Read the model definition and answer for the solid it produces. Units are mm, in the model's axes. A direction names the side the tool comes from. Give positions to 0.01 mm unless a question says otherwise; leave off trailing zeros. Write each loop counter-clockwise with the first axis right and the second up, starting at its lowest first coordinate (ties: lowest second). Pieces come first, ordered by that corner, then holes. Notation, with made-up numbers: M 58.5,35.25 L 117.5,35.25 A9 cw 117.5,46.25 Z; hole C -37.5,56.25 d7. An arc over 180 degrees is marked long. Put each result on its own line as item: value.
from build123d import *

# Parameters (mm, degrees)
SKETCH2_R           = 1.5
SKETCH2_R_2         = 33
BOSS_EXTRUDE1_DEPTH = 2
CUT_EXTRUDE1_DEPTH  = 74.566296631
FILLET1_R           = 1


with BuildPart() as part:
    # Sketch2 → Boss-Extrude1 (new body)
    with BuildSketch(Plane(origin=(0, 0, 0), x_dir=(1, 0, 0), z_dir=(0, 1, 0))):
        with BuildLine():
            Line((17.897079586, 48.929734976), (40.149284407, 43.651218265))
            ThreePointArc((40.149284407, 43.651218265), (42.540265174, 42.312242187), (43.866371506, 39.91409958))
            Line((43.866371506, 39.91409958), (49.02521675, 17.633846579))
            ThreePointArc((49.02521675, 17.633846579), (49.23478351, 16.809026698), (49.479249782, 15.993868858))
            ThreePointArc((49.479249782, 15.993868858), (51.999812242, -0.139738387), (49.392575566, -16.259565766))
            ThreePointArc((49.392575566, -16.259565766), (49.143731732, -17.073397941), (48.929734976, -17.897079586))
            Line((48.929734976, -17.897079586), (43.651218265, -40.149284407))
            ThreePointArc((43.651218265, -40.149284407), (42.312242187, -42.540265174), (39.91409958, -43.866371506))
            Line((39.91409958, -43.866371506), (17.633846579, -49.02521675))
            ThreePointArc((17.633846579, -49.02521675), (16.809026698, -49.23478351), (15.993868858, -49.479249782))
            ThreePointArc((15.993868858, -49.479249782), (-0.139738387, -51.999812242), (-16.259565766, -49.392575566))
            ThreePointArc((-16.259565766, -49.392575566), (-17.073397941, -49.143731732), (-17.897079586, -48.929734976))
            Line((-17.897079586, -48.929734976), (-40.149284407, -43.651218265))
            ThreePointArc((-40.149284407, -43.651218265), (-42.540265174, -42.312242187), (-43.866371506, -39.91409958))
            Line((-43.866371506, -39.91409958), (-49.02521675, -17.633846579))
            ThreePointArc((-49.02521675, -17.633846579), (-49.23478351, -16.809026698), (-49.479249782, -15.993868858))
            ThreePointArc((-49.479249782, -15.993868858), (-51.999812242, 0.139738387), (-49.392575566, 16.259565766))
            ThreePointArc((-49.392575566, 16.259565766), (-49.143731732, 17.073397941), (-48.929734976, 17.897079586))
            Line((-48.929734976, 17.897079586), (-43.651218265, 40.149284407))
            ThreePointArc((-43.651218265, 40.149284407), (-42.312242187, 42.540265174), (-39.91409958, 43.866371506))
            Line((-39.91409958, 43.866371506), (-17.633846579, 49.02521675))
            ThreePointArc((-17.633846579, 49.02521675), (-16.809026698, 49.23478351), (-15.993868858, 49.479249782))
            ThreePointArc((-15.993868858, 49.479249782), (-8.026622704, 51.3767781), (0.139738387, 51.999812242))
            ThreePointArc((0.139738387, 51.999812242), (8.302633013, 51.332896714), (16.259565766, 49.392575566))
            ThreePointArc((16.259565766, 49.392575566), (17.073397941, 49.143731732), (17.897079586, 48.929734976))
        make_face()
        with Locations(Location((-38.8907, 38.8907, 0), (0, 0, 270))):
            Circle(SKETCH2_R, mode=Mode.SUBTRACT)
        with Locations(Location((38.8907, 38.8907, 0), (0, 0, 90))):
            Circle(SKETCH2_R, mode=Mode.SUBTRACT)
        with Locations(Location((38.8907, -38.8907, 0), (0, 0, 270))):
            Circle(SKETCH2_R, mode=Mode.SUBTRACT)
        with Locations(Location((-38.8907, -38.8907, 0), (0, 0, 90))):
            Circle(SKETCH2_R, mode=Mode.SUBTRACT)
        with Locations(Location((0, 0, 0), (0, 0, 270))):
            Circle(SKETCH2_R_2, mode=Mode.SUBTRACT)
        with Locations(Location((0, 38.8907, 0), (0, 0, 270))):
            Circle(SKETCH2_R, mode=Mode.SUBTRACT)
        with Locations(Location((-33.680334171, -19.44535, 0), (0, 0, 270))):
            Circle(SKETCH2_R, mode=Mode.SUBTRACT)
        with Locations(Location((33.680334171, -19.44535, 0), (0, 0, 270))):
            Circle(SKETCH2_R, mode=Mode.SUBTRACT)
    extrude(amount=BOSS_EXTRUDE1_DEPTH)

    # Sketch3 → Cut-Extrude1 (cut, through all)
    with BuildSketch(Plane(origin=(0, 2, 0), x_dir=(1, 0, 0), z_dir=(0, 1, 0))):
        with BuildLine():
            Line((-21.21199112, 25.279466623), (-28.925442436, 34.47199994))
            ThreePointArc((-28.925442436, 34.47199994), (-38.97114317, 22.5), (-44.316348886, 7.814167995))
            Line((-44.316348886, 7.814167995), (-32.498655849, 5.730389863))
            ThreePointArc((-32.498655849, 5.730389863), (-28.578838325, 16.5), (-21.21199112, 25.279466623))
        make_face()
    extrude(amount=-CUT_EXTRUDE1_DEPTH, mode=Mode.SUBTRACT)

    # Fillet1
    fillet1_edges = [part.edges().sort_by_distance(p)[0] for p in [
        (-44.316348886, 1, -7.814167995),
        (-28.925442436, 1, -34.47199994),
        (-21.21199112, 1, -25.279466623),
        (-32.498655849, 1, -5.730389863),
    ]]
    fillet(fillet1_edges, radius=FILLET1_R)


solid = part.part
(1) Section A-A on z = 0 is taken. Determine the outline of the cut face in (x, y).
Result:
outline: M -52,0 L -33,0 L -33,2 L -52,2 Z; M 33,0 L 52,0 L 52,2 L 33,2 Z
(2) Section C-C on y = 0.55 is taken. Give the number of separate pieces and of enclosed holes in the cut face, and give its area (3 significant figures).
Result:
separate pieces: 1
enclosed holes: 8
area: 5,340 mm²
(3) Given pin 1 Ø1 at (y, z) = (1, -14.5) entering from +X; pin 2 Ø1 at (x, y) = (-25, 1.5) entering from -Z, each flat-ended and moving along its own axis, determine where each tip first touches the part or whether it passes through.
Result:
pin 1: stops at x = 50.08
pin 2: stops at z = -47.44
(4) Section B-B on x = 26 is taken. Determine the outline of the cut face in (y, z).
Result:
outline: M 0,-47.01 L 2,-47.01 L 2,-20.32 L 0,-20.32 Z; M 0,20.32 L 2,20.32 L 2,47.09 L 0,47.09 Z
(5) Section D-D on z = 35 is taken. Determine the outline of the cut face in (x, y).
Result:
outline: M -45,0 L 44.87,0 L 44.87,2 L -45,2 Z
(6) For a pull along Z with two mould halves and no side action, classify faces 3 (the face through (-46.327, 0.986, -28.867)), 4 (the face through (34.131, 0.986, 20.876)), 5 (the face through (-28.867, 0.986, 46.327)), 6 (the face through (-38.868, 1.014, -22.678)) as +Z half, -Z half, draft (parallel to the pull), parting line (faces both ways), or undercut.
Result:
face 3: -Z half
face 4: undercut
face 5: +Z half
face 6: undercut
(7) Which of the six approach directions +Z, -Z, +X, -X, +Y, -Y give full straight-line access (tool end or side, diameter ignored) to faces 1 (the face through (-25.015, 1.014, -29.812)), 2 (the face through (-42.34, 0.99, -42.51))?
Result:
face 1: +Y, -Y
face 2: -Z, -X, +Y, -Y
(8) Straight lines are drawn through the part: line 1 along X through (y, z) = (0.85, 40); line 2 along X through (y, z) = (0.35, 39.5); line 3 along Z through (x, y) = (-4, 0.9). For each, find the intervals that lie inside material, in ascending order. Write a range as from..to.
Result:
line 1: x = -43.85..-39.9, -37.88..37.88, 39.9..43.69
line 2: x = -43.96..-40.26, -37.52..37.52, 40.26..43.81
line 3: z = -51.85..-32.76, 32.76..51.85
